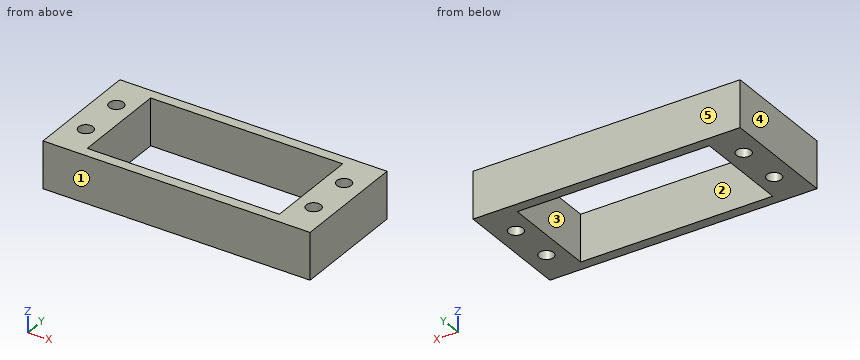
```python
from build123d import *

# Parameters (mm, degrees)
SKETCH_1_W      = 57
SKETCH_1_H      = 25
SKETCH_1_R      = 1.55
SKETCH_1_W_2    = 41
SKETCH_1_H_2    = 20.6
EXTRUDE_1_DEPTH = 10


with BuildPart() as part:
    # 草图1 → 凸台-拉伸1 (new body)
    with BuildSketch(Plane.XY):
        Rectangle(SKETCH_1_W, SKETCH_1_H)
        with Locations((24.3, 4.95)):
            Circle(SKETCH_1_R, mode=Mode.SUBTRACT)
        with Locations(Location((-24.3, 4.95, 0), (0, 0, 180))):
            Circle(SKETCH_1_R, mode=Mode.SUBTRACT)
        with Locations((-24.3, -4.95)):
            Circle(SKETCH_1_R, mode=Mode.SUBTRACT)
        with Locations(Location((24.3, -4.95, 0), (0, 0, 180))):
            Circle(SKETCH_1_R, mode=Mode.SUBTRACT)
        Rectangle(SKETCH_1_W_2, SKETCH_1_H_2, mode=Mode.SUBTRACT)
    extrude(amount=EXTRUDE_1_DEPTH)


solid = part.part
```
CAD build for the part. Positions are in the model's coordinates, mm. Face numbers are marked on the shaded views. A direction names the side the tool comes from. Round coordinates to 2 decimals unless told otherwise and drop trailing zeros. Loops run counter-clockwise (first coordinate to the right, second up) from the corner with the lowest first, then second, coordinate; pieces in that order, holes last. Notation, with made-up numbers: M 78.5,62 L 92.5,62 A24 ccw 92.5,99 Z; hole C 12,67 d4. An arc over 180 degrees is marked long. Use a Markdown table: item, result. Add a question column.
(1) Drill centre lines: line 1 (X direction, y = -5, z = 2.5); line 2 (Y direction, x = 24.3, z = 2); line 3 (X direction, y = -8.75, z = 4). Where is each one in solid material? Low to high.
(2) Cut at B-B (x = -24.3). Give the cut face in (y, z).
(3) Cut at C-C (z = 9.25). Give the cut face in (x, y).
(4) Pull direction X, two halves, no side cores. Call the marked faces 3, 4 and 5: +X half, -X half, draft (parallel to the pull), parting line (faces both ways), or undercut.
(5) Cut at D-D (y = -4.95). Give the cut face in (x, z), and give its area (3 significant figures).
(6) Which spindle directions (+Z, -Z, +X, -X, +Y, -Y) get a long thin tool onto all of the face, cutting with end or side? Do the marked faces 1 and 2. Say none if no direction does.
(7) Cut at A-A (y = -0.5). Give the cut face in (x, z), and give its area (3 significant figures).
Geometry says:
| question | item | result |
|---|---|---|
| 1 | line 1 | x = -28.5 to -25.85, -22.75 to -20.5, 20.5 to 22.75, 25.85 to 28.5 |
| 1 | line 2 | y = -12.5 to -6.5, -3.4 to 3.4, 6.5 to 12.5 |
| 1 | line 3 | x = -28.5 to -20.5, 20.5 to 28.5 |
| 2 | outline | M -12.5,0 L -6.5,0 L -6.5,10 L -12.5,10 Z; M -3.4,0 L 3.4,0 L 3.4,10 L -3.4,10 Z; M 6.5,0 L 12.5,0 L 12.5,10 L 6.5,10 Z |
| 3 | outline | M -28.5,-12.5 L 28.5,-12.5 L 28.5,12.5 L -28.5,12.5 Z; hole C -24.3,-4.95 d3.1; hole C -24.3,4.95 d3.1; hole M -20.5,-10.3 L 20.5,-10.3 L 20.5,10.3 L -20.5,10.3 Z; hole C 24.3,-4.95 d3.1; hole C 24.3,4.95 d3.1 |
| 4 | face 3 | undercut |
| 4 | face 4 | -X half |
| 4 | face 5 | draft |
| 5 | outline | M -28.5,0 L -25.85,0 L -25.85,10 L -28.5,10 Z; M -22.75,0 L -20.5,0 L -20.5,10 L -22.75,10 Z; M 20.5,0 L 22.75,0 L 22.75,10 L 20.5,10 Z; M 25.85,0 L 28.5,0 L 28.5,10 L 25.85,10 Z |
| 5 | area | 98.0 mm² |
| 6 | face 1 | +Z, -Z, +X, -X, -Y |
| 6 | face 2 | +Z, -Z |
| 7 | outline | M -28.5,0 L -20.5,0 L -20.5,10 L -28.5,10 Z; M 20.5,0 L 28.5,0 L 28.5,10 L 20.5,10 Z |
| 7 | area | 160 mm² |
